from build123d import *

# Parameters (mm, degrees)
SKIZZE1_R                       = 6.05
SKIZZE1_W                       = 4.5
SKIZZE1_H                       = 4.5
AUFSATZ_LINEAR_AUSTRAGEN1_DEPTH = 450
SKIZZE3_R                       = 3.3
SCHNITT_LINEAR_AUSTRAGEN2_DEPTH = 452.248268785


with BuildPart() as part:
    # Skizze1 → Aufsatz-Linear austragen1 (new body)
    with BuildSketch(Plane(origin=(0, 0, 0), x_dir=(-1, 0, 0), z_dir=(0, 0, -1))):
        Polygon((15.000004175, -14.999997298), (15.000004175, -3.999997298), (13.000004175, -3.999997298), (13.000004175, -7.265682298), (11.634319175, -7.265682298), (8.300003831, -3.931367382), (8.300003831, 3.931374091), (11.634315, 7.265685), (13.000004175, 7.265685), (13.000004175, 4.000002702), (15.000004175, 4.000002702), (15.000004175, 15.000002702), (4.000004175, 15.000002702), (4.000004175, 13.000002962), (7.265688438, 13.000002962), (7.265688438, 11.634318438), (3.931373306, 8.300003046), (-3.931368167, 8.300003046), (-7.265683511, 11.634317962), (-7.265683511, 13.000002962), (-3.999995825, 13.000002962), (-3.999995825, 15.000002702), (-14.999995825, 15.000002702), (-14.999995825, 4.000002702), (-12.999995825, 4.000002702), (-12.999995825, 7.265685), (-11.634315, 7.265685), (-8.3, 3.931371213), (-8.3, -3.931371213), (-11.634310825, -7.265682298), (-12.999995825, -7.265682298), (-12.999995825, -3.999997298), (-14.999995825, -3.999997298), (-14.999995825, -14.999997298), (-3.999995825, -14.999997298), (-3.999995825, -12.999997038), (-7.265683511, -12.999997038), (-7.265683511, -11.634312038), (-3.931368988, -8.299997775), (3.931373438, -8.299997775), (7.265688438, -11.634311562), (7.265688438, -12.999997038), (4.000004175, -12.999997038), (4.000004175, -14.999997298), align=None)
        with Locations(Location((0, 0, 0), (0, 0, 180))):
            Circle(SKIZZE1_R, mode=Mode.SUBTRACT)
        with Locations((11.25, 11.25)):
            Rectangle(SKIZZE1_W, SKIZZE1_H, mode=Mode.SUBTRACT)
        with Locations((11.25, -11.25)):
            Rectangle(SKIZZE1_W, SKIZZE1_H, mode=Mode.SUBTRACT)
        with Locations((-11.25, -11.25)):
            Rectangle(SKIZZE1_W, SKIZZE1_H, mode=Mode.SUBTRACT)
        with Locations((-11.25, 11.25)):
            Rectangle(SKIZZE1_W, SKIZZE1_H, mode=Mode.SUBTRACT)
    extrude(amount=-AUFSATZ_LINEAR_AUSTRAGEN1_DEPTH)

    # Skizze3 → Schnitt-Linear austragen2 (cut, through all)
    with BuildSketch(Plane.ZY.offset(15.000004175)):
        with Locations(Location((435, 0, 0), (0, 0, 180))):
            Circle(SKIZZE3_R)
        with Locations(Location((350, 0, 0), (0, 0, 180))):
            Circle(SKIZZE3_R)
    extrude(amount=-SCHNITT_LINEAR_AUSTRAGEN2_DEPTH, mode=Mode.SUBTRACT)


solid = part.part
Geometry: final body of the model. Coordinates: model frame, mm. A direction names the side the tool comes from. Give positions to 0.01 mm unless a question says otherwise; leave off trailing zeros. Write each loop counter-clockwise with the first axis right and the second up, starting at its lowest first coordinate (ties: lowest second). Pieces come first, ordered by that corner, then holes. Notation, with made-up numbers: (77, -23) -> (113, -23) arc R26 ccw to (113, 10) -> close; hole circle Ø4 at (21, -26.5). An arc over 180 degrees is marked (long way). Answer as a JSON object with one key per item and string values.
1. Ray query, probe 1 along X at (y, z) = (-12.75, 35.5); probe 2 along X at (y, z) = (-10.5, 164). Return the intervals inside material, ascending. Write a range as from..to.
Ans:
{"probe 1": "x = -15..-13.5, -9..-7.27, 7.27..9, 13.5..15", "probe 2": "x = -15..-13.5, -9..-6.13, 6.13..9, 13.5..15"}
2. Cut plane B-B on z = 375. Count the separate pieces of the cut face and the enclosed holes in it, and give its area (3 significant figures).
Ans:
{"separate pieces": "1", "enclosed holes": "5", "area": "411 mm^2"}
3. Mould query, pull axis Y, two halves, no side actions, for faces 1 (the flat face through (-8.3, 0, 222)), 2 (the flat face through (0, -8.3, 222)), 3 (the flat face through (15, 10, 222)), 4 (the flat face through (8.3, 0, 222)). Classes: pulls with the +Y half, pulls with the -Y half, needs draft (parallel to the pull), parting line crosses it, or undercut.
Ans:
{"face 1": "undercut", "face 2": "pulls with the -Y half", "face 3": "needs draft", "face 4": "undercut"}
4. Contact query for flat-ended pins moving along their axis: pin 1 (2.5 mm diameter, centred on x = -0.5, z = 272.5, fed in from +Y); pin 2 (5.5 mm diameter, centred on y = 0, z = 435, fed in from +X); pin 3 (4 mm diameter, centred on y = 0, z = 126, fed in from -X). Output: stop coordinate, or through.
Ans:
{"pin 1": "stops at y = 8.3", "pin 2": "passes through", "pin 3": "stops at x = -8.3"}
5. Cut plane A-A on x = 0. Output: boundary loops of the cut face in (y, z), and give its area (4 significant figures).
Ans:
{"outline": "(-8.3, 0) -> (-6.05, 0) -> (-6.05, 450) -> (-8.3, 450) -> close; (6.05, 0) -> (8.3, 0) -> (8.3, 450) -> (6.05, 450) -> close", "area": "2,025 mm^2"}
6. Access query for faces 5 (the flat face through (0, 8.3, 222)), 6 (the flat face through (15, -9, 222)). Directions: +Z, -Z, +X, -X, +Y, -Y. A direction counts if a zero-diameter tool reaches every point of the face in a straight line with its end or side. Return the directions, or none.
Ans:
{"face 5": "+Z, -Z, +Y", "face 6": "+Z, -Z, +X, +Y, -Y"}
